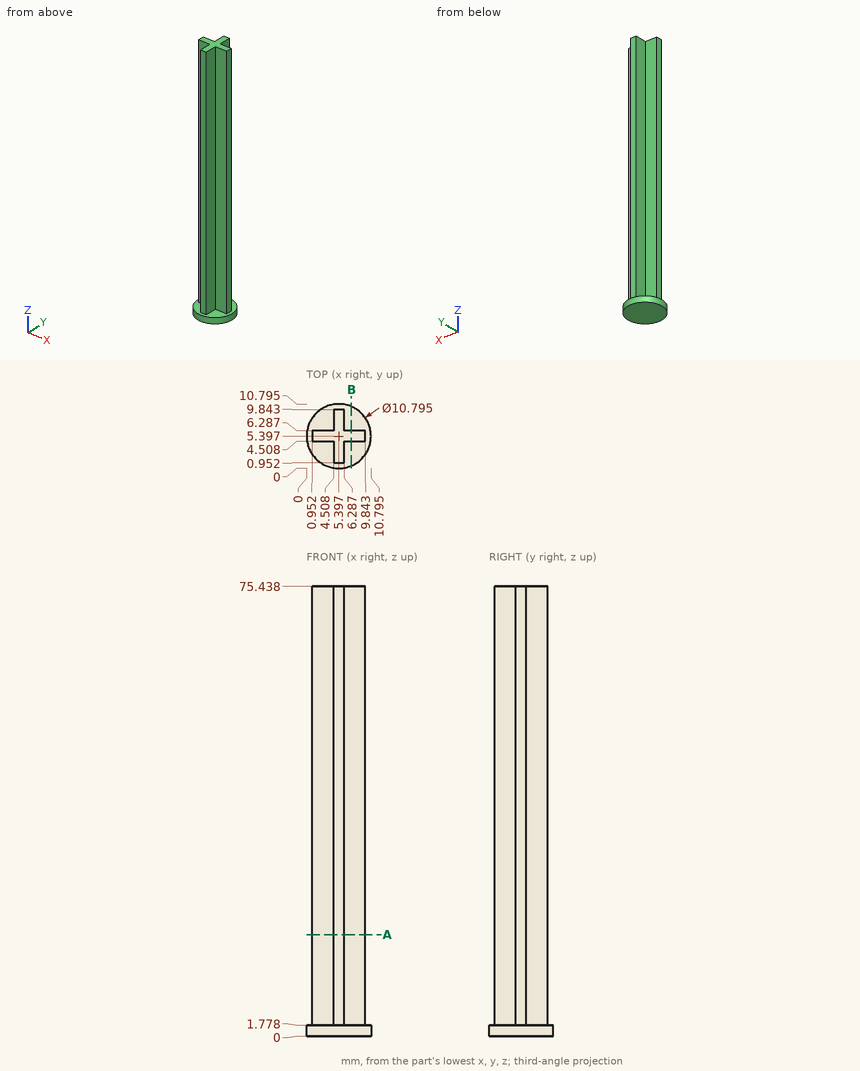
Check sheet for the drawn part. Datum: minimum x, y, z corner. Units: mm. Round coordinates to 2 decimals unless told otherwise and drop trailing zeros. Loops run counter-clockwise (first coordinate to the right, second up) from the corner with the lowest first, then second, coordinate; pieces in that order, holes last. Notation, with made-up numbers: (-4.75, -9) - (10.25, -9) arc R26 cw to (10.25, 19) - close; hole circle Ø8 at (-38.75, 64.25). An arc over 180 degrees is marked (long way). Write each question's results on one line, items separated by ' | '. Start each with the question number.
Q1. Cross-section at B-B on x = 7.5. Enter the section's corners in (y, z).
Q2. Thickness scan on line 1 (X direction, y = 1.25, z = 19); line 2 (Z direction, x = 2.25, y = 7); line 3 (Y direction, x = 4.75, z = 23). Record the ranges inside material, lowest first. Write a range as [from, to].
Q3. Cross-section at A-A on z = 17. Enter the section's corners in (x, y).
Q4. Gauge pin test, flat ends, axial feed: P1, Ø1.5, axis at x = 5.5, y = 8, coming from the -Z side; P2, Ø1.1, axis at x = 7.5, z = 28, coming from the +Y side; P3, Ø0.9, axis at y = 5.5, z = 21.5, coming from the -X side; P4, Ø0.9, axis at y = 5, z = 36.5, coming from the +X side. Record the tip position at first contact, or that the pin passes through.
Answers below:
1) outline: (0.43, 0) - (10.37, 0) - (10.37, 1.78) - (6.29, 1.78) - (6.29, 75.44) - (4.51, 75.44) - (4.51, 1.78) - (0.43, 1.78) - close
2) line 1: x = [4.51, 6.29] | line 2: z = [0, 1.78] | line 3: y = [0.95, 9.84]
3) outline: (0.95, 4.51) - (4.51, 4.51) - (4.51, 0.95) - (6.29, 0.95) - (6.29, 4.51) - (9.84, 4.51) - (9.84, 6.29) - (6.29, 6.29) - (6.29, 9.84) - (4.51, 9.84) - (4.51, 6.29) - (0.95, 6.29) - close
4) P1: stops at z = 0 | P2: stops at y = 6.29 | P3: stops at x = 0.95 | P4: stops at x = 9.84
